Geometry: see drawing. Coordinates: mm, zero at the bounding-box minimum. A direction names the side the tool comes from. Coordinates: 2 decimals unless noted, no trailing zeros. Loops run counter-clockwise (first coordinate to the right, second up) from the corner with the lowest first, then second, coordinate; pieces in that order, holes last.
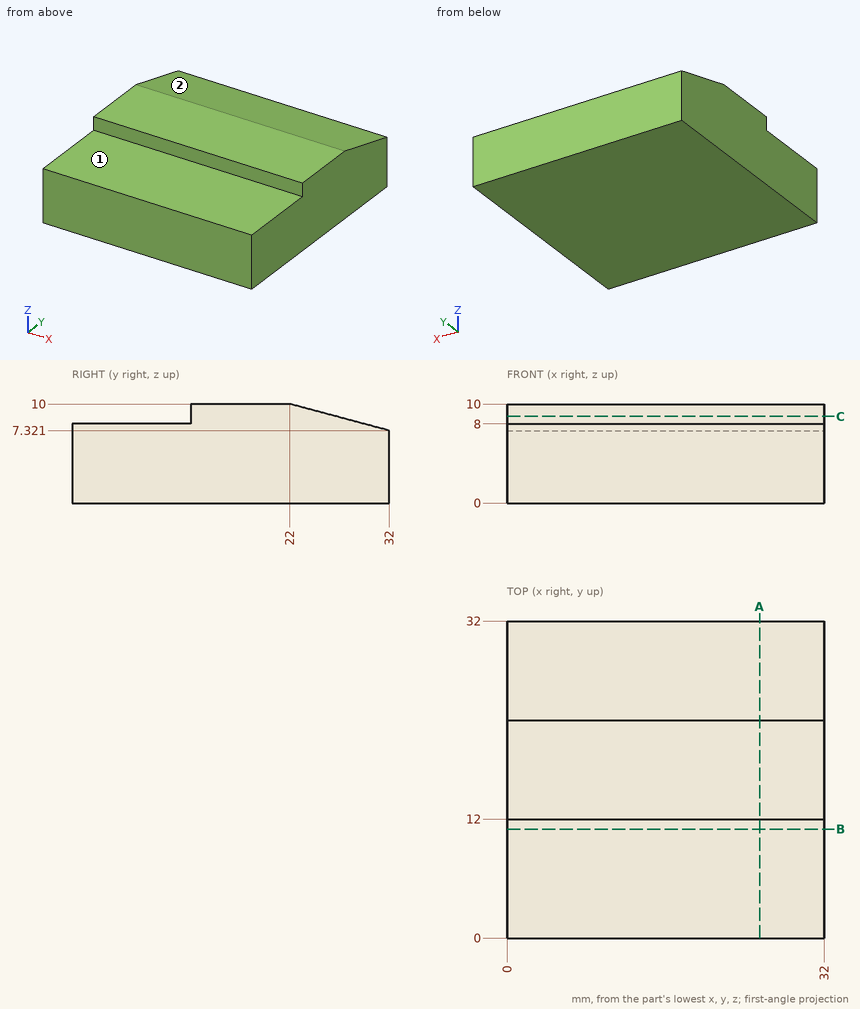
Item 1: Reachability of the marked faces 1 and 2 from +Z, -Z, +X, -X, +Y, -Y: full face, straight path, thin tool, end or side. Return the list, or none.
Result:
face 1: +Z, +X, -X, -Y
face 2: +Z, +X, -X, +Y
Item 2: Section query C-C (z = 8.75). Output: boundary loops of the cut face in (x, y) (1 decimal), then the cut area to 3 significant figures.
Result:
outline: (0, 12) - (32, 12) - (32, 26.7) - (0, 26.7) - close
area: 469 mm2
Item 3: Line query: L1, parallel to Z at x = 16, y = 11; L2, parallel to Z at x = 2.5, y = 24 (1 decimal). Output: solid intervals per line, ascending.
Result:
L1: z = 0 to 8
L2: z = 0 to 9.5
Item 4: Contact query for flat-ended pins moving along their axis: P1, Ø10, axis at x = 3, y = 9, coming from the -Z side; P2, Ø0.6, axis at x = 15.5, z = 9, coming from the -Y side. Output: stop coordinate, or through.
Result:
P1: stops at z = 0
P2: stops at y = 12
Item 5: Section query B-B (y = 11). Output: boundary loops of the cut face in (x, z), then the cut area to 3 significant figures.
Result:
outline: (0, 0) - (32, 0) - (32, 8) - (0, 8) - close
area: 256 mm2
Item 6: Section query A-A (x = 25.5). Output: boundary loops of the cut face in (y, z).
Result:
outline: (0, 0) - (32, 0) - (32, 7.32) - (22, 10) - (12, 10) - (12, 8) - (0, 8) - close
